Here's how the part is built. I have some questions about the finished solid (model axes, mm). A direction names the side the tool comes from. Give positions to 0.01 mm unless a question says otherwise; leave off trailing zeros. Write each loop counter-clockwise with the first axis right and the second up, starting at its lowest first coordinate (ties: lowest second). Pieces come first, ordered by that corner, then holes. Notation, with made-up numbers: (73, -36.5) - (132, -36.5) arc R25 cw to (132, -0.5) - close; hole circle Ø6 at (88.25, 72.25). An arc over 180 degrees is marked (long way). Use a Markdown table: item, result.
```python
from build123d import *
from build123d.topology import SkipClean

# Parameters (mm, degrees)
SKETCH_1_R          = 7.5
EXTRUDE_1_DEPTH     = 1.6
SKETCH_4_R          = 3
EXTRUDE_2_DEPTH     = 5.8
SKETCH_6_R          = 7.5
EXTRUDE_3_DEPTH     = 1.6
SKETCH_7_W          = 21
SKETCH_7_H          = 10
EXTRUDE_4_DEPTH     = 10
CHAMFER_1_SIZE      = 3
SKETCH_8_W          = 10
SKETCH_8_H          = 6
EXTRUDE_5_DEPTH     = 8
SKETCH_9_W          = 7.3
SKETCH_9_H          = 3.1
EXTRUDE_6_DEPTH     = 2.5
EXTRUDE_7_DEPTH     = 2.5
CUT_EXTRUDE_3_REACH = 50.582
SKETCH_11_R         = 1.25
CUT_EXTRUDE_4_REACH = 50.778


with BuildPart() as part:
    # 草图1 → 凸台-拉伸1 (new body)
    with BuildSketch(Plane(origin=(0, 0, 0), x_dir=(1, 0, 0), z_dir=(0, 1, 0))):
        with BuildLine():
            ThreePointArc((-2.65705645, 32.892857143), (-28.578838325, 16.5), (-29.814578114, -14.145350186))
            ThreePointArc((-29.814578114, -14.145350186), (-29.877876431, -17.25), (-27.157521664, -18.747506957))
            ThreePointArc((-27.157521664, -18.747506957), (0, -33), (27.157521664, -18.747506957))
            ThreePointArc((27.157521664, -18.747506957), (29.877876431, -17.25), (29.814578114, -14.145350186))
            ThreePointArc((29.814578114, -14.145350186), (28.578838325, 16.5), (2.65705645, 32.892857143))
            ThreePointArc((2.65705645, 32.892857143), (0, 34.5), (-2.65705645, 32.892857143))
        make_face()
        with Locations(Location((0, 0, 0), (0, 0, 270))):
            Circle(SKETCH_1_R, mode=Mode.SUBTRACT)
    extrude(amount=EXTRUDE_1_DEPTH)

    # 草图4 → 凸台-拉伸2 (add)
    with BuildSketch(Plane(origin=(0, 1.6, 0), x_dir=(1, 0, 0), z_dir=(0, 1, 0))):
        with Locations(Location((0, 31.5, 0), (0, 0, 27.664004496))):
            Circle(SKETCH_4_R)
        with Locations(Location((27.279800219, -15.75, 0), (0, 0, 32.335995504))):
            Circle(SKETCH_4_R)
        with Locations(Location((-27.279800219, -15.75, 0), (0, 0, 147.664004496))):
            Circle(SKETCH_4_R)
    extrude(amount=EXTRUDE_2_DEPTH)

    # 草图6 → 凸台-拉伸3 (add)
    with SkipClean():  # the faces are left unmerged after this step: merging them gives an invalid solid
        with BuildSketch(Plane(origin=(0, 7.4, 0), x_dir=(1, 0, 0), z_dir=(0, 1, 0))):
            with BuildLine():
                Line((-21, -14), (21, -14))
                Line((21, -14), (25.210881382, -21.293460498))
                ThreePointArc((25.210881382, -21.293460498), (26.215126916, -20.044129334), (27.157521664, -18.747506957))
                ThreePointArc((27.157521664, -18.747506957), (29.877876431, -17.25), (29.814578114, -14.145350186))
                ThreePointArc((29.814578114, -14.145350186), (28.578838325, 16.5), (2.65705645, 32.892857143))
                ThreePointArc((2.65705645, 32.892857143), (0, 34.5), (-2.65705645, 32.892857143))
                ThreePointArc((-2.65705645, 32.892857143), (-28.578838325, 16.5), (-29.814578114, -14.145350186))
                ThreePointArc((-29.814578114, -14.145350186), (-29.877876431, -17.25), (-27.157521664, -18.747506957))
                ThreePointArc((-27.157521664, -18.747506957), (-26.215126916, -20.044129334), (-25.210881382, -21.293460498))
                Line((-25.210881382, -21.293460498), (-21, -14))
            make_face()
            with Locations(Location((0, 0, 0), (0, 0, 270))):
                Circle(SKETCH_6_R, mode=Mode.SUBTRACT)
        extrude(amount=EXTRUDE_3_DEPTH)

    # 草图7 → 凸台-拉伸4 (add)
    with SkipClean():  # the faces are left unmerged after this step: merging them gives an invalid solid
        with BuildSketch(Plane(origin=(0, 1.6, 0), x_dir=(1, 0, 0), z_dir=(0, 1, 0))):
            with Locations((0, -22)):
                Rectangle(SKETCH_7_W, SKETCH_7_H)
        extrude(amount=EXTRUDE_4_DEPTH)

    # 倒角1
    chamfer_1_edges = [part.edges().sort_by_distance(p)[0] for p in [
        (0, 11.6, 17),
        (0, 11.6, 27),
    ]]
    chamfer(chamfer_1_edges, length=CHAMFER_1_SIZE)

    # 草图8 → 凸台-拉伸5 (add)
    with SkipClean():  # the faces are left unmerged after this step: merging them gives an invalid solid
        with BuildSketch(Plane(origin=(0, 1.6, 0), x_dir=(1, 0, 0), z_dir=(0, 1, 0))):
            with Locations((-16.5, -21)):
                Rectangle(SKETCH_8_W, SKETCH_8_H)
        extrude(amount=EXTRUDE_5_DEPTH)

    # 草图9 → 凸台-拉伸6 (add)
    with SkipClean():  # the faces are left unmerged after this step: merging them gives an invalid solid
        with BuildSketch(Plane(origin=(0, 9, 0), x_dir=(1, 0, 0), z_dir=(0, 1, 0))):
            with Locations((4, -10.632060859)):
                Rectangle(SKETCH_9_W, SKETCH_9_H)
        extrude(amount=EXTRUDE_6_DEPTH)

    # 草图10 → 凸台-拉伸7 (add)
    with SkipClean():  # the faces are left unmerged after this step: merging them gives an invalid solid
        with BuildSketch(Plane(origin=(0, 9, 0), x_dir=(1, 0, 0), z_dir=(0, 1, 0))):
            Polygon((-13.835733856, 24.945439837), (-3.469217829, 28.313725076), (-4.612580708, 31.832634186), (-14.979096735, 28.464348947), align=None)
        extrude(amount=EXTRUDE_7_DEPTH)

    # 草图11 → 切除-拉伸3 (cut, up to next)
    with BuildSketch(Plane(origin=(0, 9, 0), x_dir=(1, 0, 0), z_dir=(0, 1, 0)), mode=Mode.PRIVATE) as cut_extrude_3_sk1:
        with Locations(Location((0, 31.5, 0), (0, 0, 270))):
            Circle(SKETCH_11_R)
    cut_extrude_3_tool1 = extrude(cut_extrude_3_sk1.sketch, amount=-CUT_EXTRUDE_3_REACH, mode=Mode.PRIVATE) & part.part
    # 草图11 → 切除-拉伸3 (cut, up to next)
    with BuildSketch(Plane(origin=(0, 9, 0), x_dir=(1, 0, 0), z_dir=(0, 1, 0)), mode=Mode.PRIVATE) as cut_extrude_3_sk2:
        with Locations(Location((27.279800219, -15.75, 0), (0, 0, 270))):
            Circle(SKETCH_11_R)
    cut_extrude_3_tool2 = extrude(cut_extrude_3_sk2.sketch, amount=-CUT_EXTRUDE_3_REACH, mode=Mode.PRIVATE) & part.part
    # 草图11 → 切除-拉伸3 (cut, up to next)
    with BuildSketch(Plane(origin=(0, 9, 0), x_dir=(1, 0, 0), z_dir=(0, 1, 0)), mode=Mode.PRIVATE) as cut_extrude_3_sk3:
        with Locations(Location((-27.279800219, -15.75, 0), (0, 0, 270))):
            Circle(SKETCH_11_R)
    cut_extrude_3_tool3 = extrude(cut_extrude_3_sk3.sketch, amount=-CUT_EXTRUDE_3_REACH, mode=Mode.PRIVATE) & part.part
    add(cut_extrude_3_tool1.solids().sort_by_distance((0, 9, -31.5))[0], mode=Mode.SUBTRACT)
    add(cut_extrude_3_tool2.solids().sort_by_distance((27.2798, 9, 15.75))[0], mode=Mode.SUBTRACT)
    add(cut_extrude_3_tool3.solids().sort_by_distance((-27.2798, 9, 15.75))[0], mode=Mode.SUBTRACT)

    # 草图12 → 切除-拉伸4 (cut, up to next)
    with BuildSketch(Plane(origin=(0, 1.6, 0), x_dir=(1, 0, 0), z_dir=(0, 1, 0)), mode=Mode.PRIVATE) as cut_extrude_4_sk1:
        with BuildLine():
            Line((18.973665961, -27), (-18.973665961, -27))
            ThreePointArc((-18.973665961, -27), (0, -33), (18.973665961, -27))
        make_face()
    cut_extrude_4_tool1 = extrude(cut_extrude_4_sk1.sketch, amount=-CUT_EXTRUDE_4_REACH, mode=Mode.PRIVATE) & part.part
    add(cut_extrude_4_tool1.solids().sort_by_distance((0, 1.6, 29.419743))[0], mode=Mode.SUBTRACT)


solid = part.part
```
Item 1: If we section it at A-A, the plane y = 10.5: Write out the boundary of the cut face in (x, z).
Values:
| item | result |
|---|---|
| outline | (-14.98, -28.46) - (-4.61, -31.83) - (-3.47, -28.31) - (-13.84, -24.95) - close; (-10.5, 18.9) - (10.5, 18.9) - (10.5, 25.1) - (-10.5, 25.1) - close; (0.35, 9.08) - (7.65, 9.08) - (7.65, 12.18) - (0.35, 12.18) - close |
Item 2: Thinking about a two-plate mould opening in X: for faces 5 (the flat face through (7, 0, -4)), 6 (the cylindrical face through (28.8, 8.19, -16.11)), 7 (the flat face through (-14.415, 10.232, -26.73)), 8 (the cylindrical face through (26.06, 4.56, 15.48)), which applies, +X half, -X half, draft (parallel to the pull), parting line (faces both ways), or undercut?
Values:
| item | result |
|---|---|
| face 5 | draft |
| face 6 | +X half |
| face 7 | -X half |
| face 8 | undercut |
Item 3: For faces 1 (the flat face through (-8.725, 10.232, -26.606)), 2 (the flat face through (7.65, 10, 11)), 3 (the flat face through (-17, 6, 24)), 4 (the flat face through (-11.5, 6, 21)), which set-ups out of +Z, -Z, +X, -X, +Y, -Y let a thin tool reach every point of the face, with its end or its side?
Values:
| item | result |
|---|---|
| face 1 | +X, +Y |
| face 2 | -Z, +X, +Y |
| face 3 | +Z, -X, +Y |
| face 4 | +Z, +Y |
Item 4: If we section it at D-D, the plane z = -1: Write out the boundary of the cut face in (x, y).
Values:
| item | result |
|---|---|
| outline | (-32.98, 0) - (-7.43, 0) - (-7.43, 1.6) - (-32.98, 1.6) - close; (-32.98, 7.4) - (-7.43, 7.4) - (-7.43, 9) - (-32.98, 9) - close; (7.43, 0) - (32.98, 0) - (32.98, 1.6) - (7.43, 1.6) - close; (7.43, 7.4) - (32.98, 7.4) - (32.98, 9) - (7.43, 9) - close |
Item 5: If we section it at B-B, the plane z = 15.75: Write out the boundary of the cut face in (x, y), plus the area to 3 significant figures.
Values:
| item | result |
|---|---|
| outline | (-30.28, 0) - (-28.53, 0) - (-28.53, 9) - (-30.28, 9) - close; (-26.03, 0) - (26.03, 0) - (26.03, 9) - (22.01, 9) - (22.01, 7.4) - (24.28, 7.4) - (24.28, 1.6) - (-24.28, 1.6) - (-24.28, 7.4) - (-22.01, 7.4) - (-22.01, 9) - (-26.03, 9) - close; (28.53, 0) - (30.28, 0) - (30.28, 9) - (28.53, 9) - close |
| area | 148 mm2 |
Item 6: Will these pins go through, and if not, where does the flat tip stop? pin 1 Ø3 at (x, y) = (15, 9.5) entering from -Z; pin 2 Ø3 at (y, z) = (9.5, 10.5) entering from -X; pin 3 Ø4 at (x, z) = (-11, -21.5) entering from +Y; pin 4 Ø4 at (x, z) = (-27.28, 15.75) entering from -Y.
Values:
| item | result |
|---|---|
| pin 1 | stops at z = -30.07 |
| pin 2 | stops at x = -31.72 |
| pin 3 | stops at y = 9 |
| pin 4 | stops at y = 0 |
Item 7: If we section it at C-C, the plane x = 4: Write out the boundary of the cut face in (y, z).
Values:
| item | result |
|---|---|
| outline | (0, -32.76) - (1.6, -32.76) - (1.6, -6.34) - (0, -6.34) - close; (0, 6.34) - (1.6, 6.34) - (1.6, 17) - (8.6, 17) - (11.6, 20) - (11.6, 24) - (8.6, 27) - (0, 27) - close; (7.4, -32.76) - (9, -32.76) - (9, -6.34) - (7.4, -6.34) - close; (7.4, 6.34) - (9, 6.34) - (9, 9.08) - (11.5, 9.08) - (11.5, 12.18) - (9, 12.18) - (9, 14) - (7.4, 14) - close |
Item 8: I need wall thicknesses on line 1 along X through (y, z) = (4.75, 15.75); line 2 along Y through (x, z) = (14, 8.5); line 3 along X through (y, z) = (8.25, 16). Which ranges of each line are inside material? Lowest first, please. Write a range as [from, to].
Values:
| item | result |
|---|---|
| line 1 | x = [-30.28, -28.53], [-26.03, -24.28], [24.28, 26.03], [28.53, 30.28] |
| line 2 | y = [0, 1.6], [7.4, 9] |
| line 3 | x = [-30.27, -28.5], [-26.06, -22.15], [22.15, 26.06], [28.5, 30.27] |
